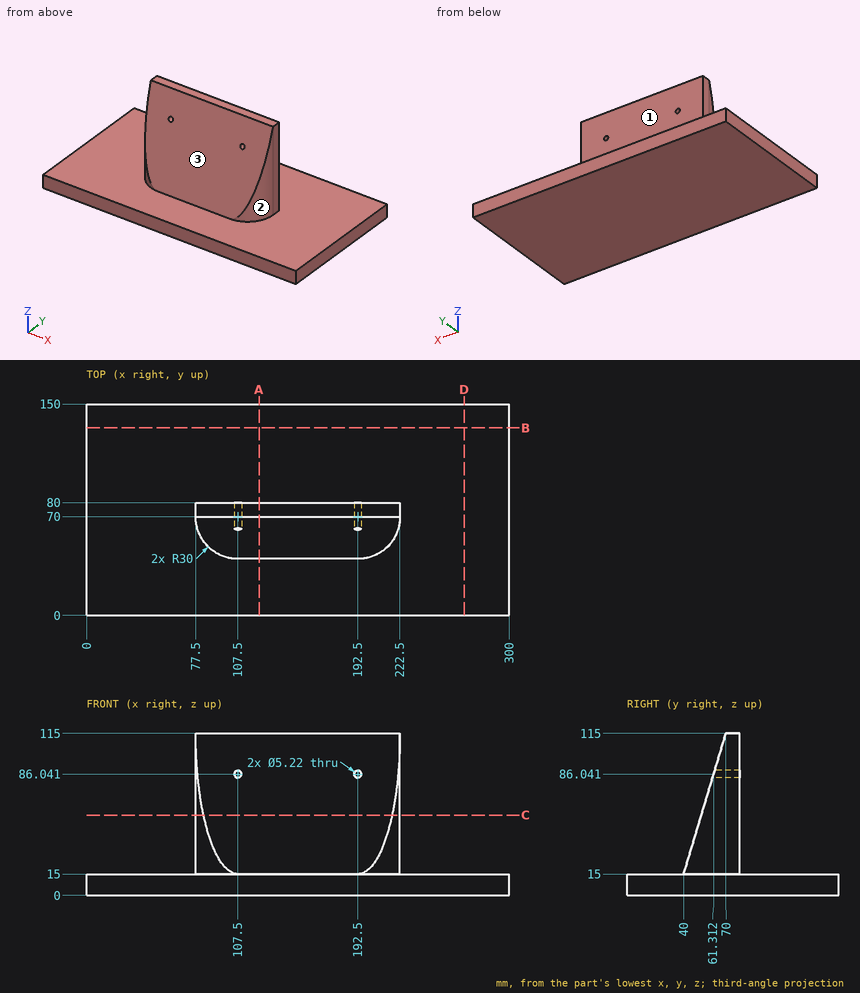
For this review, use the dimensioned drawing (mm, ordinates from the lowest corner) and the shaded views. A direction names the side the tool comes from. Round coordinates to 2 decimals unless told otherwise and drop trailing zeros. Order: outer loops, then holes, each group sorted by start corner. A loop starts at its lowest first (then second) coordinate and runs counter-clockwise, first axis right, second up. Notation, with made-up numbers: (-34, 19) -> (11, 19) arc R29 ccw to (11, 45) -> close; hole circle Ø11 at (0, -6). An arc over 180 degrees is marked (long way). Put each result on its own line as item: value.
Q1. Add section C-C on z = 57. Write out the cut boundary in (x, y).
Check result:
outline: (77.5, 70) arc R30 ccw to (83.06, 52.6) -> (216.94, 52.6) arc R30 ccw to (222.5, 70) -> (222.5, 80) -> (77.5, 80) -> close
Q2. For probe 1 along X at (y, z) = (70.5, 36); probe 2 along Z at (x, y) = (220, 88); probe 3 along X at (y, z) = (68, 83), list the stretches that pass through material, from the lowest coordinate up. Write a range as [from, to].
Check result:
probe 1: [77.5, 222.5]
probe 2: [0, 15]
probe 3: [77.57, 222.43]
Q3. Insertion check: pin 1 Ø5 at (y, z) = (73.5, 43.5) entering from +X; pin 2 Ø4 at (x, z) = (192.5, 86.04) entering from -Y; pin 3 Ø8 at (x, z) = (178, 53) entering from +Y; pin 4 Ø3 at (y, z) = (76.5, 77) entering from -X. Each pin has a flat end and moves straight along its axis. Give the tip position at first contact, or say it passes through.
Check result:
pin 1: x = 222.5
pin 2: through
pin 3: y = 80
pin 4: x = 77.5
Q4. Add section A-A on x = 122.5. Write out the cut boundary in (y, z), plus the area to 3 significant figures.
Check result:
outline: (0, 0) -> (150, 0) -> (150, 15) -> (80, 15) -> (80, 115) -> (70, 115) -> (40, 15) -> (0, 15) -> close
area: 4,750 mm2
Q5. Add section B-B on y = 133. Write out the cut boundary in (x, z), plus the area to 3 significant figures.
Check result:
outline: (0, 0) -> (300, 0) -> (300, 15) -> (0, 15) -> close
area: 4,500 mm2
Q6. Machinability: for the marked faces 1, 2 and 3, which of the approach directions +Z, -Z, +X, -X, +Y, -Y give a long, thin tool a straight path to every point of the face, cutting with its end or side? Answer none if there is none.
Check result:
face 1: +Z, +X, -X, +Y
face 2: +Z, +X, -Y
face 3: +Z, +X, -X, -Y
Q7. Add section D-D on x = 268. Write out the cut boundary in (y, z).
Check result:
outline: (0, 0) -> (150, 0) -> (150, 15) -> (0, 15) -> close
